Could you check a few things on this model? Use its own coordinates, in mm. Face numbers are marked on the shaded views. Coordinates: 2 decimals unless noted, no trailing zeros. Order: outer loops, then holes, each group sorted by start corner. A loop starts at its lowest first (then second) coordinate and runs counter-clockwise, first axis right, second up. Notation, with made-up numbers: (68, -8) - (106, -8) arc R32 ccw to (106, 26) - close; hole circle Ø8 at (25, 70.25). An arc over 180 degrees is marked (long way). One line per item, written item: value.
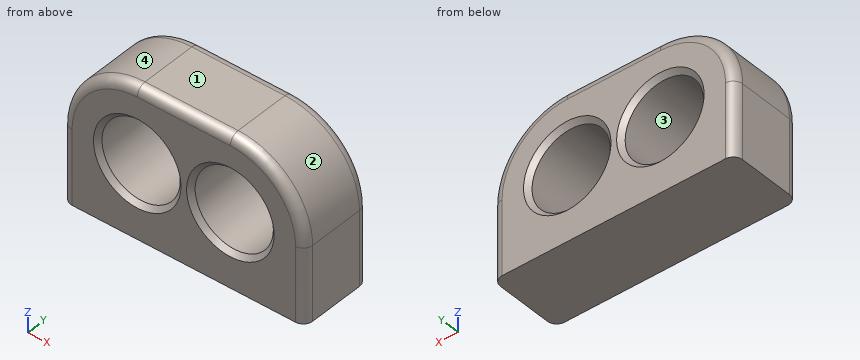
Solid Edge part; units mm, degrees
sketch "Sketch1" plane through (0, 0, 0) normal (0, -1, 0) x (1, 0, 0)
  circle A0 centre (0, 0) radius 2.1
  circle A1 centre (-5, 0) radius 2.1
  line L0 (-5, 4) -> (0, 4)
  line L1 (4, -4) -> (4, 0)
  line L2 (0, -4) -> (4, -4)
  line L3 (-5, -4) -> (0, -4)
  line L4 (-9, -4) -> (-5, -4)
  line L5 (-9, 0) -> (-9, -4)
  arc A2 (-9, 0) -> (-5, 4) centre (-5, 0) cw
  arc A3 (0, 4) -> (4, 0) centre (0, 0) cw
extrude "Protrusion1" add sketch "Sketch1" along normal mid plane 4
fillet "Verrundung_1" radius 0.5 10 edges at (-2.5, -2, 4) (2.8284, -2, 2.8284) (4, -2, -2) (-7.8284, -2, 2.8284) (-9, -2, -2) (2.8284, 2, 2.8284) (4, 2, -2) (-2.5, 2, 4) (-7.8284, 2, 2.8284) (-9, 2, -2)
chamfer "Fase_1" distance 0.25 angle 45 4 edges at (-7.1, -2, 0) (-7.1, 2, 0) (-2.1, -2, 0) (-2.1, 2, 0)
properties part number "086" material "PLA"
Item 1: Thinking about a two-plate mould opening in X: for the marked faces 1, 2, 3 and 4, which applies, pulls with the +X half, pulls with the -X half, needs draft (parallel to the pull), parting line crosses it, or undercut?
Conclusion:
face 1: needs draft
face 2: pulls with the +X half
face 3: undercut
face 4: pulls with the -X half
Item 2: If I drill on probe 1 along Z at (x, y) = (-5, 1); probe 2 along Z at (x, y) = (-3.5, 1.1); probe 3 along Z at (x, y) = (3, -1.3), over which ranges is the centre line in solid material (lowest first)?
Conclusion:
probe 1: -4 to -2.1, 2.1 to 4
probe 2: -4 to -1.47, 1.47 to 4
probe 3: -4 to 2.65
Item 3: I want a section at A-A on y = -1. Please give me the cut outline in (x, z).
Conclusion:
outline: (-9, -4) - (4, -4) - (4, 0) arc R4 ccw to (0, 4) - (-5, 4) arc R4 ccw to (-9, 0) - close; hole circle Ø4.2 at (-5, 0); hole circle Ø4.2 at (0, 0)
Item 4: I want a section at B-B on z = 1. Give the number of separate pieces and of enclosed holes in the cut face, then the cut area to 3 significant figures.
Conclusion:
separate pieces: 3
enclosed holes: 0
area: 20.9 mm²
